Build history of the part. All positions in model axes, mm. Face numbers are marked on the shaded views. A direction names the side the tool comes from. Round coordinates to 2 decimals unless told otherwise and drop trailing zeros. Write each loop counter-clockwise with the first axis right and the second up, starting at its lowest first coordinate (ties: lowest second). Pieces come first, ordered by that corner, then holes. Notation, with made-up numbers: (31, 87) -> (75, 87) arc R16 ccw to (75, 113) -> close; hole circle Ø9 at (76.5, -19). An arc over 180 degrees is marked (long way). Answer in a Markdown table with one row per item. Add a question column.
from build123d import *

# Parameters (mm, degrees)
EXTRUDE_1_DEPTH        = 27
CUT_EXTRUDE_1_REACH    = 29
SKETCH_3_W             = 1
SKETCH_3_H             = 7
SKETCH_8_W             = 12.8
SKETCH_8_H             = 27
CUT_EXTRUDE_4_DEPTH    = 1.9
CUT_EXTRUDE_5_REACH    = 29
SKETCH_9_R             = 1.15
SKETCH_9_W             = 6.8
SKETCH_9_H             = 1.3
CUT_EXTRUDE_START      = -27
SKETCH_11_W            = 3.1
SKETCH_11_H            = 1
CUT_EXTRUDE_6_DEPTH    = 27
FILLET_1_R             = 2
FILLET_2_R             = 0.2
HOLE_WIZARD_M3_1_D     = 2.5
HOLE_WIZARD_M3_1_DEPTH = 8.5
HOLE_WIZARD_M3_1_TIP   = 0.751075774


with BuildPart() as part:
    # 草图1 → 凸台-拉伸1 (new body)
    with BuildSketch(Plane(origin=(0, 0, 0), x_dir=(1, 0, 0), z_dir=(0, 1, 0))):
        Polygon((-9.5, 11.35), (-9.5, 0), (9.5, 0), (9.5, 11.35), (5.1, 11.35), (5.1, 8.35), (6.4, 8.35), (6.4, 2.3), (-6.4, 2.3), (-6.4, 8.35), (-5.1, 8.35), (-5.1, 11.35), align=None)
    extrude(amount=EXTRUDE_1_DEPTH)

    # 草图3 → 切除-拉伸1 (cut, up to next)
    with BuildSketch(Plane(origin=(0, 27, 0), x_dir=(1, 0, 0), z_dir=(0, 1, 0)), mode=Mode.PRIVATE) as cut_extrude_1_sk1:
        with Locations((-8, 7.85)):
            Rectangle(SKETCH_3_W, SKETCH_3_H)
    cut_extrude_1_tool1 = extrude(cut_extrude_1_sk1.sketch, amount=-CUT_EXTRUDE_1_REACH, mode=Mode.PRIVATE) & part.part
    add(cut_extrude_1_tool1.solids().sort_by_distance((-8, 27, -7.85))[0], mode=Mode.SUBTRACT)
    # 草图3 → 切除-拉伸1 (cut, up to next)
    with BuildSketch(Plane(origin=(0, 27, 0), x_dir=(1, 0, 0), z_dir=(0, 1, 0)), mode=Mode.PRIVATE) as cut_extrude_1_sk2:
        with Locations((8, 7.85)):
            Rectangle(SKETCH_3_W, SKETCH_3_H)
    cut_extrude_1_tool2 = extrude(cut_extrude_1_sk2.sketch, amount=-CUT_EXTRUDE_1_REACH, mode=Mode.PRIVATE) & part.part
    add(cut_extrude_1_tool2.solids().sort_by_distance((8, 27, -7.85))[0], mode=Mode.SUBTRACT)

    # 草图8 → 切除-拉伸4 (cut)
    with BuildSketch(Plane(origin=(0, 0, -11.35), x_dir=(-1, 0, 0), z_dir=(0, 0, -1))):
        with Locations((0, 13.5)):
            Rectangle(SKETCH_8_W, SKETCH_8_H)
    extrude(amount=-CUT_EXTRUDE_4_DEPTH, mode=Mode.SUBTRACT)

    # 草图9 → 切除-拉伸5 (cut, up to next)
    with BuildSketch(Plane.XZ, mode=Mode.PRIVATE) as cut_extrude_5_sk1:
        with Locations((-6.4, -2.3)):
            Circle(SKETCH_9_R)
    cut_extrude_5_tool1 = extrude(cut_extrude_5_sk1.sketch, amount=-CUT_EXTRUDE_5_REACH, mode=Mode.PRIVATE) & part.part
    add(cut_extrude_5_tool1.solids().sort_by_distance((-6.4, 0, -2.3))[0], mode=Mode.SUBTRACT)
    # 草图9 → 切除-拉伸5 (cut, up to next)
    with BuildSketch(Plane.XZ, mode=Mode.PRIVATE) as cut_extrude_5_sk2:
        with Locations((6.4, -2.3)):
            Circle(SKETCH_9_R)
    cut_extrude_5_tool2 = extrude(cut_extrude_5_sk2.sketch, amount=-CUT_EXTRUDE_5_REACH, mode=Mode.PRIVATE) & part.part
    add(cut_extrude_5_tool2.solids().sort_by_distance((6.4, 0, -2.3))[0], mode=Mode.SUBTRACT)
    # 草图9 → 切除-拉伸5 (cut, up to next)
    with BuildSketch(Plane.XZ, mode=Mode.PRIVATE) as cut_extrude_5_sk3:
        with Locations((0, -1.65)):
            Rectangle(SKETCH_9_W, SKETCH_9_H)
    cut_extrude_5_tool3 = extrude(cut_extrude_5_sk3.sketch, amount=-CUT_EXTRUDE_5_REACH, mode=Mode.PRIVATE) & part.part
    add(cut_extrude_5_tool3.solids().sort_by_distance((0, 0, -1.65))[0], mode=Mode.SUBTRACT)

    # 草图11 → 切除-拉伸6 (cut)
    with BuildSketch(Plane(origin=(0, 27, 0), x_dir=(1, 0, 0), z_dir=(0, 1, 0)).offset(CUT_EXTRUDE_START)):
        with Locations((7.95, 10.85)):
            Rectangle(SKETCH_11_W, SKETCH_11_H)
        with Locations((-7.95, 10.85)):
            Rectangle(SKETCH_11_W, SKETCH_11_H)
    extrude(amount=CUT_EXTRUDE_6_DEPTH, mode=Mode.SUBTRACT)

    # 圆角1
    fillet_1_edges = [part.edges().sort_by_distance(p)[0] for p in [
        (9.5, 13.5, 0),
        (-9.5, 13.5, 0),
    ]]
    fillet(fillet_1_edges, radius=FILLET_1_R)

    # 圆角2
    fillet_2_edges = [part.edges().sort_by_distance(p)[0] for p in [
        (-3.4, 13.5, -2.3),
        (-3.4, 13.5, -1),
        (3.4, 13.5, -1),
        (3.4, 13.5, -2.3),
        (9.5, 13.5, -10.35),
        (-9.5, 13.5, -10.35),
        (6.4, 13.5, -10.35),
        (-6.4, 13.5, -10.35),
        (-5.1, 13.5, -8.35),
        (5.1, 13.5, -8.35),
        (5.1, 13.5, -9.45),
        (-5.1, 13.5, -9.45),
    ]]
    fillet(fillet_2_edges, radius=FILLET_2_R)

    # M3 螺纹孔1
    with Locations(Plane(origin=(0, 27, 0), x_dir=(1, 0, 0), z_dir=(0, 1, 0))):
        with Locations((-6.4, 2.3), (6.4, 2.3)):
            Hole(HOLE_WIZARD_M3_1_D / 2, depth=HOLE_WIZARD_M3_1_DEPTH)
            with Locations((0, 0, -(HOLE_WIZARD_M3_1_DEPTH + HOLE_WIZARD_M3_1_TIP / 2))):  # 118° drill point
                Cone(0, HOLE_WIZARD_M3_1_D / 2, HOLE_WIZARD_M3_1_TIP, mode=Mode.SUBTRACT)


solid = part.part
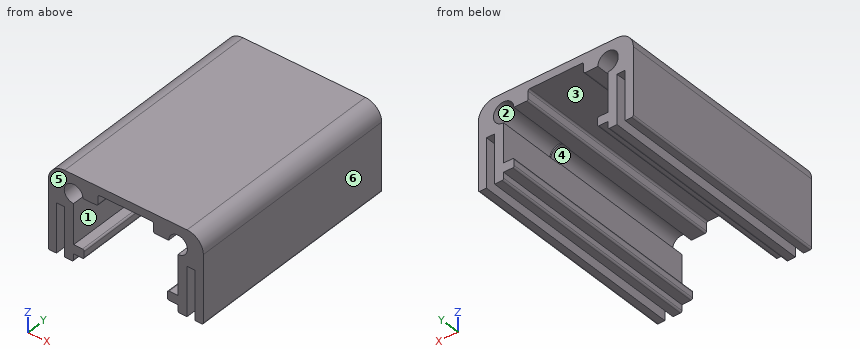
(1) Saw through at A-A (z = -7). List the corners of the cut face in (x, y).
(2) Saw through at C-C (x = 0). List the corners of the cut face in (y, z), plus the area to 3 significant figures.
(3) Which spindle directions (+Z, -Z, +X, -X, +Y, -Y) get a long thin tool onto all of the face, cutting with end or side? Do the marked faces 1, 2 and 3. Say none if no direction does.
(4) Probe line 1 along X through (y, z) = (2.5, -5); line 2 along Z through (x, y) = (6.75, 2.5); line 3 along Z through (x, y) = (1.25, 4.5). List the from-to ranges inside material, lowest first.
(5) Drop flat-ended pins along their axis: P1, Ø1.9, axis at x = -0.5, y = 11, coming from the -Z side; P2, Ø0.5, axis at x = 4.5, y = 10, coming from the -Z side; P3, Ø1.8, axis at x = 6.4, z = -2.3, coming from the +Y side. Give the stop position or say it passes through.
(6) Mould opens along X. For the marked faces 4, 5 and 6 say: pulls with the +X half, pulls with the -X half, needs draft (parallel to the pull), parting line crosses it, or undercut.
(7) Saw through at B-B (z = -4). List the corners of the cut face in (x, y).
Answer sheet:
| question | item | result |
|---|---|---|
| 1 | outline | (-9.5, 0) -> (-8.5, 0) -> (-8.5, 27) -> (-9.5, 27) -> close; (-7.5, 0) -> (-6.4, 0) -> (-6.4, 27) -> (-7.5, 27) -> close; (6.4, 0) -> (7.5, 0) -> (7.5, 27) -> (6.4, 27) -> close; (8.5, 0) -> (9.5, 0) -> (9.5, 27) -> (8.5, 27) -> close |
| 2 | outline | (0, -1) -> (27, -1) -> (27, 0) -> (0, 0) -> close |
| 2 | area | 27.0 mm² |
| 3 | face 1 | +Y, -Y |
| 3 | face 2 | +Y |
| 3 | face 3 | -Z, +Y, -Y |
| 4 | line 1 | x = -9.5 to -8.5, -7.5 to -6.4, 6.4 to 7.5, 8.5 to 9.5 |
| 4 | line 2 | z = -10.35 to -3.4, -1.2 to 0 |
| 4 | line 3 | z = -1 to 0 |
| 5 | P1 | stops at z = -1 |
| 5 | P2 | stops at z = -2.3 |
| 5 | P3 | passes through |
| 6 | face 4 | undercut |
| 6 | face 5 | needs draft |
| 6 | face 6 | pulls with the +X half |
| 7 | outline | (-9.5, 0) -> (-6.4, 0) -> (-6.4, 27) -> (-9.5, 27) -> close; (6.4, 0) -> (9.5, 0) -> (9.5, 27) -> (6.4, 27) -> close |
